from build123d import *

# Parameters (mm, degrees)
ESBO_O1_W                                            = 450
ESBO_O1_H                                            = 150
RESSALTO_EXTRUS_O1_DEPTH                             = 40
REBAIXO_PARA_PARAFUSO_ALLEN_SEXTAVADO_DE_D           = 11
REBAIXO_PARA_PARAFUSO_ALLEN_SEXTAVADO_DE_DEPTH       = 40
REBAIXO_PARA_PARAFUSO_ALLEN_SEXTAVADO_DE_CBORE_D     = 18
REBAIXO_PARA_PARAFUSO_ALLEN_SEXTAVADO_DE_CBORE_DEPTH = 7.1
FURO_ROSCADO_DE_M18X2_0_D                            = 16
FURO_ROSCADO_DE_M18X2_0_DEPTH                        = 40


with BuildPart() as part:
    # Esboço1 → Ressalto-extrusão1 (new body)
    with BuildSketch(Plane(origin=(0, 0, 0), x_dir=(1, 0, 0), z_dir=(0, 1, 0))):
        Rectangle(ESBO_O1_W, ESBO_O1_H)
    extrude(amount=RESSALTO_EXTRUS_O1_DEPTH)

    # Rebaixo para parafuso Allen sextavado de M101
    with Locations(Plane(origin=(0, 40, 0), x_dir=(1, 0, 0), z_dir=(0, 1, 0))):
        with Locations((-200, 50), (-100, 50), (0, 50), (100, 50), (200, 50), (-100, -50), (0, -50), (100, -50), (200, -50), (-200, -50)):
            CounterBoreHole(REBAIXO_PARA_PARAFUSO_ALLEN_SEXTAVADO_DE_D / 2, REBAIXO_PARA_PARAFUSO_ALLEN_SEXTAVADO_DE_CBORE_D / 2, REBAIXO_PARA_PARAFUSO_ALLEN_SEXTAVADO_DE_CBORE_DEPTH, depth=REBAIXO_PARA_PARAFUSO_ALLEN_SEXTAVADO_DE_DEPTH)

    # Furo roscado de M18x2.0
    with Locations(Plane(origin=(0, 40, 0), x_dir=(1, 0, 0), z_dir=(0, 1, 0))):
        with Locations((0, 0), (150, 0), (-150, 0)):
            Hole(FURO_ROSCADO_DE_M18X2_0_D / 2, depth=FURO_ROSCADO_DE_M18X2_0_DEPTH)


solid = part.part
Input: part model. Units: mm. Frame: model coordinates. A direction names the side the tool comes from. Round coordinates to 2 decimals unless told otherwise and drop trailing zeros. Write each loop counter-clockwise with the first axis right and the second up, starting at its lowest first coordinate (ties: lowest second). Pieces come first, ordered by that corner, then holes.
1) Cut plane B-B (y = 27). Count the separate pieces of the cut face and the enclosed holes in it, then the cut area to 3 significant figures.
2) Contact query for flat-ended pins moving along their axis: P1, Ø14.5, axis at x = 200, z = 50, coming from the -Y side; P2, Ø9, axis at x = 101.5, z = 50, coming from the +Y side. Output: stop coordinate, or through.
3) Cut plane D-D (x = -200). Return the cut outline in (y, z).
4) Cut plane C-C (z = 0). Return the cut outline in (x, y).
5) Ray query, L1, parallel to Z at x = 200, y = 35; L2, parallel to X at y = 21, z = 50; L3, parallel to X at y = 38, z = -50. Return the intervals inside material, ascending.
6) Draft query along Z for faces 1 (the flat face through (-3, 0, -18)), 2 (the flat face through (-4, 32.9, -46)), 3 (the flat face through (-3, 20, 75)). Return one class per face: pulls with the +Z half, pulls with the -Z half, needs draft (parallel to the pull), parting line crosses it, or undercut.
7) Reachability of faces 4 (the flat face through (-3, 20, -75)), 5 (the flat face through (-4, 32.9, 54)) from +Z, -Z, +X, -X, +Y, -Y: full face, straight path, thin tool, end or side. Return the list, or none.
8) Cut plane A-A (x = 150). Return the cut outline in (y, z), then the cut area to 3 significant figures.
Geometry says:
1. separate pieces: 1
1. enclosed holes: 13
1. area: 65,900 mm2
2. P1: stops at y = 0
2. P2: stops at y = 32.9
3. outline: (0, -75) - (40, -75) - (40, -59) - (32.9, -59) - (32.9, -55.5) - (0, -55.5) - close; (0, -44.5) - (32.9, -44.5) - (32.9, -41) - (40, -41) - (40, 41) - (32.9, 41) - (32.9, 44.5) - (0, 44.5) - close; (0, 55.5) - (32.9, 55.5) - (32.9, 59) - (40, 59) - (40, 75) - (0, 75) - close
4. outline: (-225, 0) - (-158, 0) - (-158, 40) - (-225, 40) - close; (-142, 0) - (-8, 0) - (-8, 40) - (-142, 40) - close; (8, 0) - (142, 0) - (142, 40) - (8, 40) - close; (158, 0) - (225, 0) - (225, 40) - (158, 40) - close
5. L1: z = -75 to -59, -41 to 41, 59 to 75
5. L2: x = -225 to -205.5, -194.5 to -105.5, -94.5 to -5.5, 5.5 to 94.5, 105.5 to 194.5, 205.5 to 225
5. L3: x = -225 to -209, -191 to -109, -91 to -9, 9 to 91, 109 to 191, 209 to 225
6. face 1: needs draft
6. face 2: undercut
6. face 3: pulls with the +Z half
7. face 4: -Z, +X, -X, +Y, -Y
7. face 5: +Y
8. outline: (0, -75) - (40, -75) - (40, -8) - (0, -8) - close; (0, 8) - (40, 8) - (40, 75) - (0, 75) - close
8. area: 5,360 mm2
